For this review, take the finished solid that the model builds, in its own axes (mm). A direction names the side the tool comes from. Round coordinates to 2 decimals unless told otherwise and drop trailing zeros. Order: outer loops, then holes, each group sorted by start corner. A loop starts at its lowest first (then second) coordinate and runs counter-clockwise, first axis right, second up. Notation, with made-up numbers: M 47.25,86.5 L 62.25,86.5 A5 cw 62.25,94.5 Z; hole C 51,34.25 d8. An arc over 180 degrees is marked long. Answer as a JSON object with one key per item and string values.
Autodesk Inventor part; units mm, degrees
ref_plane "YZ Plane" through (0, 0, 0) normal (1, 0, 0) x (0, 1, 0)
ref_plane "XZ Plane" through (0, 0, 0) normal (0, 1, 0) x (-1, 0, 0)
ref_plane "XY Plane" through (0, 0, 0) normal (0, 0, 1) x (1, 0, 0)
sketch "Sketch1" plane through (0, 0, 0) normal (0, 1, 0) x (-1, 0, 0)
  line L0 (0, 0) -> (-59, 0)
  line L1 (-59, 0) -> (-59, 5)
  line L2 (-59, 5) -> (0, 5)
  line L3 (0, 5) -> (0, 0)
  line L4 (0, 5) -> (-5, 5)
  line L5 (-5, 5) -> (-5, 47)
  line L6 (-5, 47) -> (0, 47)
  line L7 (0, 47) -> (0, 5)
  line L8 (-59, 5) -> (-54, 5)
  line L9 (-54, 5) -> (-54, 47)
  line L10 (-54, 47) -> (-59, 47)
  line L11 (-59, 47) -> (-59, 5)
  point P0 (-54, 5)
  dimension "d0" = 59
  dimension "d1" = 5
  dimension "d2" = 5
  dimension "d3" = 42
  dimension "d4" = 5
  dimension "d5" = 42
extrude "Extrusion1" add sketch "Sketch1" against normal blind 62
sketch "Sketch7" plane through (0, -62, 0) normal (0, -1, 0) x (1, 0, 0)
  line L0 (0, 47) -> (0, 0)
  line L1 (0, 47) -> (-5, 47)
  line L2 (-5, 47) -> (-5, -5)
  line L3 (-5, -5) -> (0, -5)
  line L4 (0, -5) -> (0, 47)
  line L5 (59, 47) -> (54, 47)
  line L6 (59, 47) -> (64, 47)
  line L7 (64, 47) -> (64, -5)
  line L8 (64, -5) -> (59, -5)
  line L9 (59, -5) -> (59, 47)
  line L10 (0, 0) -> (59, 0)
  line L11 (59, -5) -> (0, -5)
  line L12 (0, -5) -> (0, 0)
  line L13 (0, 0) -> (59, 0)
  line L14 (59, 0) -> (59, -5)
  dimension "d34" = 5
  dimension "d35" = 52
  dimension "d36" = 5
  dimension "d37" = 52
extrude "Extrusion7" add sketch "Sketch7" against normal blind 8
sketch "Sketch8" plane through (0, -62, 0) normal (0, -1, 0) x (1, 0, 0)
  line L0 (0, 0) -> (0, 47)
  line L1 (5, 47) -> (-5, 47)
  circle A0 centre (0, 37) radius 2.6
  line L2 (59, 47) -> (59, 0)
  line L3 (64, 47) -> (54, 47)
  circle A1 centre (59, 37) radius 2.6
  line L4 (59, 0) -> (0, 0)
  line L5 (-5, 47) -> (-5, -5)
  line L6 (64, -5) -> (64, 47)
  circle A2 centre (16.5, 0) radius 2.6
  circle A3 centre (42.5, 0) radius 2.6
  point P0 (29.5, 0)
  dimension "d40" = 10
  dimension "d41" = 5.2
  dimension "d42" = 10
  dimension "d43" = 5.2
  dimension "d44" = 34.5
  dimension "d47" = 5.2
  dimension "d48" = 5.2
  dimension "d56" = 13
  dimension "d57" = 13
extrude "Extrusion8" cut sketch "Sketch8" against normal blind 5
sketch "Sketch9" plane through (0, 0, 0) normal (-1, 0, 0) x (0, 0, 1)
  point P0 (0, 0)
sketch "Sketch10" plane through (0, 0, 0) normal (-1, 0, 0) x (0, 0, 1)
  line L0 (47, 0) -> (47, -54)
  line L1 (47, -62) -> (-5, -62)
  circle A0 centre (26, -12) radius 3
  point P0 (0, 0)
  dimension "d51" = 21
  dimension "d52" = 50
  dimension "d53" = 6
extrude "Extrusion9" cut sketch "Sketch10" against normal blind 5
equation "\"d4\" = d2"
equation "\"d5\" = d3"
equation "\"d43\" = d41"
equation "\"d47\" = d41"
equation "\"d48\" = d47"
properties part number "top cam mount v04"
1) Add section B-B on y = -12. State the section outline as (x, z) points.
Geometry check:
{"outline": "M 0,0 L 59,0 L 59,47 L 54,47 L 54,5 L 5,5 L 5,23 L 0,23 Z; M 0,29 L 5,29 L 5,47 L 0,47 Z"}
2) Add section C-C on x = 42.5. State the section outline as (y, z) points, and give its area (3 significant figures).
Geometry check:
{"outline": "M -62,-5 L -54,-5 L -54,0 L 0,0 L 0,5 L -62,5 L -62,2.6 L -57,2.6 L -57,-2.6 L -62,-2.6 Z", "area": "324 mm²"}
3) For L1, parallel to X at y = -58.3, z = 37; L2, parallel to X at y = -14, z = 40.5; L3, parallel to Z at x = 59, y = -59, list the stretches that pass through material, from the lowest coordinate up.
Geometry check:
{"L1": "x = -5 to -2.6, 2.6 to 5, 54 to 56.4, 61.6 to 64", "L2": "x = 0 to 5, 54 to 59", "L3": "z = -5 to 34.4, 39.6 to 47"}
4) Mouldability with a two-part tool opening along Z and no side actions: class faces 1 (the flat face through (-5, -58, 21)), 2 (the flat face through (59, -57, 37)), 3 (the flat face through (29, -58, -5)) as +Z half, -Z half, draft (parallel to the pull), parting line (faces both ways), or undercut.
Geometry check:
{"face 1": "draft", "face 2": "undercut", "face 3": "-Z half"}
5) Add section A-A on z = 20. State the section outline as (x, y) points, and give its area (3 significant figures).
Geometry check:
{"outline": "M -5,-62 L 5,-62 L 5,0 L 0,0 L 0,-54 L -5,-54 Z; M 54,-62 L 64,-62 L 64,-54 L 59,-54 L 59,0 L 54,0 Z", "area": "700 mm²"}
6) Machinability: for faces 4 (the flat face through (59, -27, 23)), 5 (the flat face through (0, -27, 24)), 6 (the flat face through (16, -57, 0)), which of the approach directions +Z, -Z, +X, -X, +Y, -Y give a long, thin tool a straight path to every point of the face, cutting with its end or side? Answer none if there is none.
Geometry check:
{"face 4": "+Z, -Z, +X, +Y", "face 5": "+Z, -Z, -X, +Y", "face 6": "-Y"}
7) Add section D-D on z = 27.5. State the section outline as (x, y) points.
Geometry check:
{"outline": "M -5,-62 L 5,-62 L 5,-14.6 L 0,-14.6 L 0,-54 L -5,-54 Z; M 0,-9.4 L 5,-9.4 L 5,0 L 0,0 Z; M 54,-62 L 64,-62 L 64,-54 L 59,-54 L 59,0 L 54,0 Z"}
8) Insertion check: P1, Ø4.5, axis at x = 16.5, z = 0, coming from the +Y side; P2, Ø12.5, axis at y = -29.5, z = 18.5, coming from the +X side; P3, Ø4, axis at x = 59, z = 37, coming from the -Y side; P4, Ø5, axis at y = -12, z = 26, coming from the -X side. Each pin has a flat end and moves straight along its axis. Give the tip position at first contact, or say it passes through.
Geometry check:
{"P1": "stops at y = 0", "P2": "stops at x = 59", "P3": "stops at y = -57", "P4": "stops at x = 54"}
